Could you check a few things on this drawing? It's one solid part, dimensions in mm from its lowest x, y, z. A direction names the side the tool comes from. Coordinates: 2 decimals unless noted, no trailing zeros. Write each loop counter-clockwise with the first axis right and the second up, starting at its lowest first coordinate (ties: lowest second). Pieces come first, ordered by that corner, then holes.
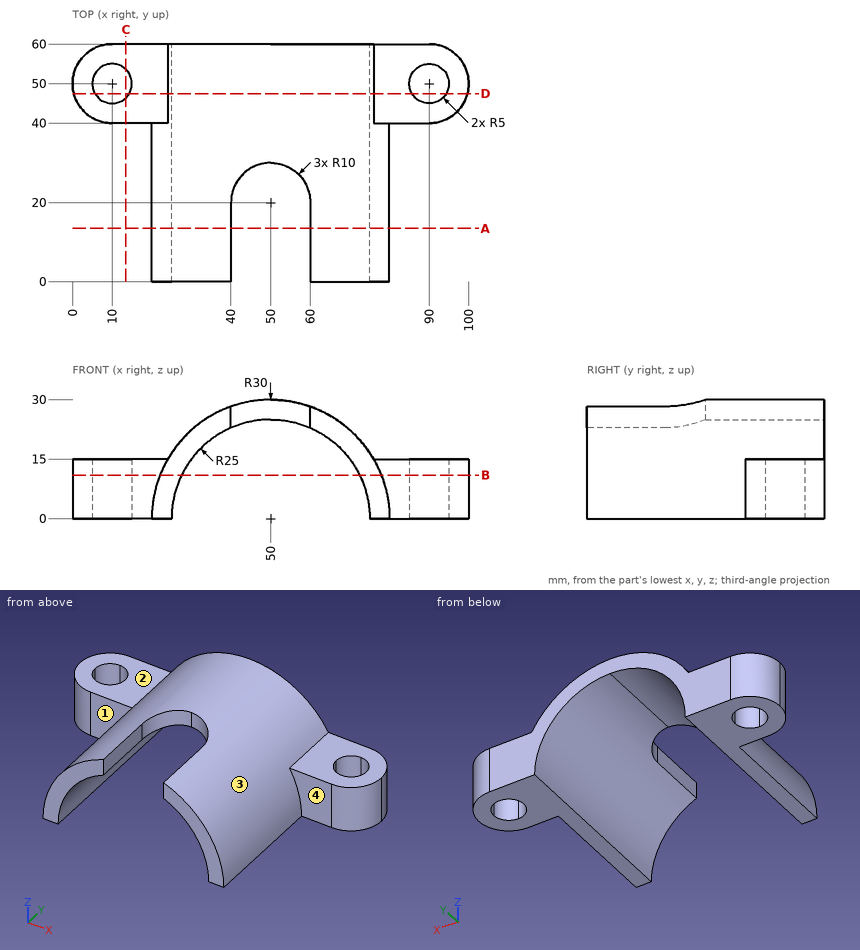
1) Imagine slicing it at B-B on z = 11. Please give me the cut outline in (x, y).
Values follow:
outline: (10, 40) - (22.09, 40) - (22.09, 0) - (27.55, 0) - (27.55, 60) - (10, 60) arc R10 ccw to start; (72.45, 0) - (77.91, 0) - (77.91, 40) - (90, 40) arc R10 ccw to (90, 60) - (72.45, 60) - close; hole circle Ø10 at (10, 50); hole circle Ø10 at (90, 50)
2) On a 3-axis mill with a long thin cutter (end or side, diameter ignored), from which of +Z, -Z, +X, -X, +Y, -Y can I reach the whole of each face in a straight line? I mean the marked faces 1, 2, 3 and 4. Say none if no direction works.
Values follow:
face 1: +Z, -X, -Y
face 2: +Z, -X, +Y, -Y
face 3: +Z, -Y
face 4: +Z, +X, -Y
3) I need wall thicknesses on probe 1 along X at (y, z) = (54, 7); probe 2 along X at (y, z) = (52, 3.5); probe 3 along X at (y, z) = (32.5, 7.5). Which ranges of each line are inside material? Lowest first, please.
Values follow:
probe 1: x = 0.83 to 7, 13 to 26, 74 to 87, 93 to 99.17
probe 2: x = 0.2 to 5.42, 14.58 to 25.25, 74.75 to 85.42, 94.58 to 99.8
probe 3: x = 20.95 to 26.15, 73.85 to 79.05
4) Imagine slicing it at C-C on x = 13.5. Please give me the cut outline in (y, z).
Values follow:
outline: (40, 0) - (46.43, 0) - (46.43, 15) - (40, 15) - close; (53.57, 0) - (60, 0) - (60, 15) - (53.57, 15) - close
5) Imagine slicing it at A-A on y = 13.5. Please give me the cut outline in (x, z).
Values follow:
outline: (20, 0) - (25, 0) arc R25 cw to (40, 22.91) - (40, 28.28) arc R30 ccw to start; (60, 22.91) arc R25 cw to (75, 0) - (80, 0) arc R30 ccw to (60, 28.28) - close
6) Imagine slicing it at D-D on y = 47.5. Please give me the cut outline in (x, z), then the cut area to 3 significant figures.
Values follow:
outline: (0.32, 0) - (5.67, 0) - (5.67, 15) - (0.32, 15) - close; (14.33, 0) - (25, 0) arc R25 cw to (75, 0) - (85.67, 0) - (85.67, 15) - (75.98, 15) arc R30 ccw to (24.02, 15) - (14.33, 15) - close; (94.33, 0) - (99.68, 0) - (99.68, 15) - (94.33, 15) - close
area: 802 mm2
7) Will these pins go through, and if not, where does the flat tip stop? pin 1 (4.5 mm diameter, centred on y = 9.5, z = 27, fed in from +X); pin 2 (8 mm diameter, centred on y = 17, z = 25.5, fed in from -X); pin 3 (6 mm diameter, centred on y = 15, z = 15, fed in from -X).
Values follow:
pin 1: stops at x = 66.95
pin 2: stops at x = 29.08
pin 3: stops at x = 22.5
